```python
from build123d import *

# Parameters (mm, degrees)
SKIZZE1_W                       = 25.4
SKIZZE1_H                       = 128.5
AUFSATZ_LINEAR_AUSTRAGEN1_DEPTH = 3
SCHNITT_LINEAR_AUSTRAGEN4_DEPTH = 4
SKIZZE3_R                       = 3.15
SCHNITT_LINEAR_AUSTRAGEN6_DEPTH = 4


with BuildPart() as part:
    # Skizze1 → Aufsatz-Linear austragen1 (new body)
    with BuildSketch(Plane(origin=(0, 0, 0), x_dir=(1, 0, 0), z_dir=(0, 1, 0))):
        Rectangle(SKIZZE1_W, SKIZZE1_H)
    extrude(amount=AUFSATZ_LINEAR_AUSTRAGEN1_DEPTH)

    # Skizze2 → Schnitt-Linear austragen4 (cut, through all)
    with BuildSketch(Plane(origin=(0, 0, 0), x_dir=(1, 0, 0), z_dir=(0, 1, 0))):
        with BuildLine():
            Line((-5.2, 62.85), (-2.2, 62.85))
            ThreePointArc((-2.2, 62.85), (-0.6, 61.25), (-2.2, 59.65))
            Line((-2.2, 59.65), (-5.2, 59.65))
            ThreePointArc((-5.2, 59.65), (-6.8, 61.25), (-5.2, 62.85))
        make_face()
        with BuildLine():
            Line((-5.2, -59.65), (-2.2, -59.65))
            ThreePointArc((-2.2, -59.65), (-0.6, -61.25), (-2.2, -62.85))
            Line((-2.2, -62.85), (-5.2, -62.85))
            ThreePointArc((-5.2, -62.85), (-6.8, -61.25), (-5.2, -59.65))
        make_face()
    extrude(amount=SCHNITT_LINEAR_AUSTRAGEN4_DEPTH, mode=Mode.SUBTRACT)

    # Skizze3 → Schnitt-Linear austragen6 (cut, through all)
    with BuildSketch(Plane(origin=(0, 0, 0), x_dir=(1, 0, 0), z_dir=(0, 1, 0))):
        with Locations((0.7, -44.25)):
            Circle(SKIZZE3_R)
        with Locations((0.7, -34.25)):
            Circle(SKIZZE3_R)
        with Locations((0.7, -24.25)):
            Circle(SKIZZE3_R)
        with Locations((0.7, -14.25)):
            Circle(SKIZZE3_R)
        with Locations((0.7, -4.25)):
            Circle(SKIZZE3_R)
        with Locations((0.7, 5.75)):
            Circle(SKIZZE3_R)
        with Locations((0.7, 15.75)):
            Circle(SKIZZE3_R)
        with Locations((0.7, 25.75)):
            Circle(SKIZZE3_R)
    extrude(amount=SCHNITT_LINEAR_AUSTRAGEN6_DEPTH, mode=Mode.SUBTRACT)


solid = part.part
```
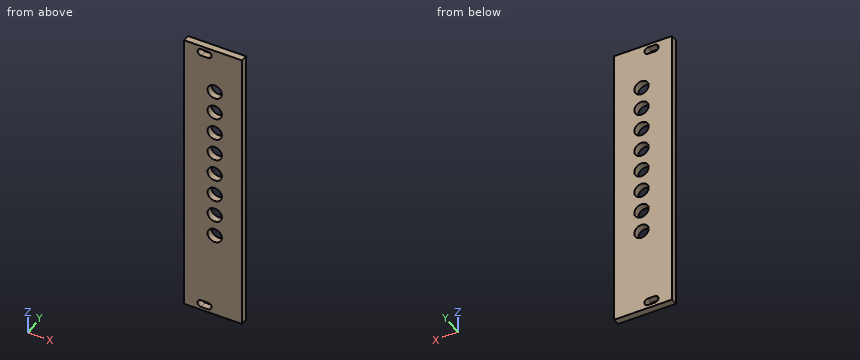
Could you check a few things on this model? Use its own coordinates, in mm. Round coordinates to 2 decimals unless told otherwise and drop trailing zeros. Loops run counter-clockwise (first coordinate to the right, second up) from the corner with the lowest first, then second, coordinate; pieces in that order, holes last. Notation, with made-up numbers: (49, 53.5) - (72, 53.5) arc R15 cw to (72, 65.5) - close; hole circle Ø4 at (21, 82.25). An arc over 180 degrees is marked (long way). Use CSV: the item, a comma, the result in double quotes.
Item 1: If we section it at D-D on z = 14.25: List the corners of the cut face in (x, y) for me, then the cut area to 3 significant figures.
Here are the results:
outline,"(-12.7, 0) - (-2.45, 0) - (-2.45, 3) - (-12.7, 3) - close; (3.85, 0) - (12.7, 0) - (12.7, 3) - (3.85, 3) - close"
area,"57.3 mm²"
Item 2: If we section it at A-A on z = -61.25: List the corners of the cut face in (x, y) for me, then the cut area to 3 significant figures.
Here are the results:
outline,"(-12.7, 0) - (-6.8, 0) - (-6.8, 3) - (-12.7, 3) - close; (-0.6, 0) - (12.7, 0) - (12.7, 3) - (-0.6, 3) - close"
area,"57.6 mm²"
Item 3: I need wall thicknesses on L1, parallel to X at y = 1.45, z = -26; L2, parallel to X at y = 0.7, z = 23. Which ranges of each line are inside material? Lowest first, please. Write a range as [from, to].
Here are the results:
L1,"x = [-12.7, -2.44], [3.84, 12.7]"
L2,"x = [-12.7, -2.19], [3.59, 12.7]"
Item 4: If we section it at B-B on y = 0.9: Count the separate pieces of the cut face and the enclosed holes in it, then the cut area to 3 significant figures.
Here are the results:
separate pieces,"1"
enclosed holes,"10"
area,"2,980 mm²"
